The model under review builds one solid part; all positions refer to its coordinate system, in mm. A direction names the side the tool comes from. Coordinates: 2 decimals unless noted, no trailing zeros. Order: outer loops, then holes, each group sorted by start corner. A loop starts at its lowest first (then second) coordinate and runs counter-clockwise, first axis right, second up. Notation, with made-up numbers: (-0.75, 50) -> (16.25, 50) arc R28 ccw to (16.25, 74) -> close; hole circle Ø7 at (47, -18). An arc over 180 degrees is marked (long way). Use one line per item in the form item = value. Start each with the question number.
(1) Take a section at D-D (y = 3.75). State the section outline as (x, z) points.
(2) For faces 5 (the flat face through (0, 4.75, -19)), 6 (the flat face through (2.715, 9.521, -15.653)), 7 (the cylindrical face through (16.39, 10.1, -17.49)), list the 3-axis set-ups (+Z, -Z, +X, -X, +Y, -Y) from which the entire face can be reached by the end or side of a thin tool; tool diameter is ignored.
(3) Take a section at B-B (z = -27.25). State the section outline as (x, y) points.
(4) Insertion check: pin 1 Ø3.5 at (x, z) = (0, -17.25) entering from -Y; pin 2 Ø4 at (x, z) = (0, -17.25) entering from -Y; pin 3 Ø3.5 at (x, y) = (-10, -3.75) entering from +Z. Each pin has a flat end and moves straight along its axis. Give the tip position at first contact, or say it passes through.
(5) Wall thickness on line 1 along Y through (x, z) = (4, -18.5); line 2 along Y through (x, z) = (-2, -27.25); line 3 along Y through (x, z) = (-14.5, -22): over which ranges is each line inside the solid? List them lowest first.
(6) Mouldability with a two-part tool opening along Y and no side actions: class faces 1 (the cylindrical face through (0.241, 3.632, -30.248)), 2 (the flat face through (0, 0, -34.5)), 3 (the flat face through (2, 8, -17)), 4 (the cylindrical face through (-16.35, -10.14, -17.49)) as +Y half, -Y half, draft (parallel to the pull), parting line (faces both ways), or undercut.
(7) Take a section at A-A (x = -10). State the section outline as (y, z) points, then the cut area to 3 significant figures.
(8) Take a section at C-C (x = 0). State how many separate pieces and enclosed holes the cut face has, then the cut area to 3 significant figures.
```python
from build123d import *

# Parameters (mm, degrees)
SKETCH1_W           = 34.5
SKETCH1_H           = 22
BOSS_EXTRUDE1_DEPTH = 34.5
SKETCH2_R           = 3
CUT_EXTRUDE1_DEPTH  = 51.014997751
SKETCH3_R           = 1.5
CUT_EXTRUDE2_DEPTH  = 3
SKETCH3_3_R         = 1.5
CUT_EXTRUDE3_DEPTH  = 45.405095428
CHAMFER1_SIZE       = 2
FILLET1_R           = 3


with BuildPart() as part:
    # Sketch1 → Boss-Extrude1 (new body)
    with BuildSketch(Plane.XY):
        Rectangle(SKETCH1_W, SKETCH1_H)
        with BuildLine():
            ThreePointArc((-7.171572875, -4.75), (-13, -3.75), (-7.171572875, -2.75))
            Line((-7.171572875, -2.75), (7.171572875, -2.75))
            ThreePointArc((7.171572875, -2.75), (10.507305936, -0.793204321), (13, -3.75))
            ThreePointArc((13, -3.75), (10.507305936, -6.706795679), (7.171572875, -4.75))
            Line((7.171572875, -4.75), (-7.171572875, -4.75))
        make_face(mode=Mode.SUBTRACT)
    extrude(amount=-BOSS_EXTRUDE1_DEPTH)

    # Sketch2 → Cut-Extrude1 (cut, through all)
    with BuildSketch(Plane(origin=(17.25, 0, 0), x_dir=(0, 0, -1), z_dir=(1, 0, 0))):
        with Locations((7.25, 3.75)):
            Circle(SKETCH2_R)
        with BuildLine():
            Line((10.078427125, 2.75), (24.421572875, 2.75))
            ThreePointArc((24.421572875, 2.75), (24.25, 3.75), (24.421572875, 4.75))
            Line((24.421572875, 4.75), (10.078427125, 4.75))
            ThreePointArc((10.078427125, 4.75), (10.206795679, 4.257305936), (10.25, 3.75))
            ThreePointArc((10.25, 3.75), (10.206795679, 3.242694064), (10.078427125, 2.75))
        make_face()
        with Locations((27.25, 3.75)):
            Circle(SKETCH2_R)
    extrude(amount=-CUT_EXTRUDE1_DEPTH, mode=Mode.SUBTRACT)

    # Sketch3 → Cut-Extrude2 (cut)
    # profile 1 of 2: a face of its own
    with BuildSketch(Plane(origin=(0, 11, 0), x_dir=(1, 0, 0), z_dir=(0, 1, 0))):
        Polygon((3.637306696, 17.25), (1.818653348, 20.4), (-1.818653348, 20.4), (-3.637306696, 17.25), (-1.818653348, 14.1), (1.818653348, 14.1), align=None)
        with Locations((0, 17.25)):
            Circle(SKETCH3_R, mode=Mode.SUBTRACT)
    # profile 2 of 2: a face of its own
    with BuildSketch(Plane(origin=(0, 11, 0), x_dir=(1, 0, 0), z_dir=(0, 1, 0))):
        with Locations((0, 17.25)):
            Circle(SKETCH3_R)
    extrude(amount=-CUT_EXTRUDE2_DEPTH, mode=Mode.SUBTRACT)

    # Sketch3_3 → Cut-Extrude3 (cut, through all)
    with BuildSketch(Plane(origin=(0, 11, 0), x_dir=(1, 0, 0), z_dir=(0, 1, 0))):
        with Locations(Location((0, 17.25, 0), (0, 0, 270))):
            Circle(SKETCH3_3_R)
    extrude(amount=-CUT_EXTRUDE3_DEPTH, mode=Mode.SUBTRACT)

    # Chamfer1
    chamfer1_edges = [part.edges().sort_by_distance(p)[0] for p in [
        (0, -11, -18.75),
    ]]
    chamfer(chamfer1_edges, length=CHAMFER1_SIZE)

    # Fillet1
    fillet1_edges = [part.edges().sort_by_distance(p)[0] for p in [
        (17.25, -11, -17.25),
        (-17.25, -11, -17.25),
        (-17.25, 11, -17.25),
        (17.25, 11, -17.25),
    ]]
    fillet(fillet1_edges, radius=FILLET1_R)


solid = part.part
```
Findings:
q1.outline = (-17.25, -34.5) -> (17.25, -34.5) -> (17.25, -30.25) -> (-17.25, -30.25) -> close; (-17.25, -4.25) -> (17.25, -4.25) -> (17.25, 0) -> (-17.25, 0) -> close
q2.face_5 = +X, -X
q2.face_6 = +Y
q2.face_7 = +Z, -Z, +X, +Y
q3.outline = (-17.25, -8) arc R3 ccw to (-14.25, -11) -> (14.25, -11) arc R3 ccw to (17.25, -8) -> (17.25, 0.75) -> (-17.25, 0.75) -> close; (-17.25, 6.75) -> (17.25, 6.75) -> (17.25, 8) arc R3 ccw to (14.25, 11) -> (-14.25, 11) arc R3 ccw to (-17.25, 8) -> close; hole (-7.17, -4.75) -> (7.17, -4.75) arc R3 ccw (long way) to (7.17, -2.75) -> (-7.17, -2.75) arc R3 ccw (long way) to start
q4.pin_1 = -9.25
q4.pin_2 = -9.5
q4.pin_3 = through
q5.line_1 = -11 to -4.75, -2.75 to 2.75, 4.75 to 11
q5.line_2 = -11 to -4.75, -2.75 to 0.75, 6.75 to 11
q5.line_3 = -10.99 to 2.75, 4.75 to 10.99
q6.face_1 = undercut
q6.face_2 = draft
q6.face_3 = +Y half
q6.face_4 = -Y half
q7.outline = (-11, -34.5) -> (-6.75, -34.5) -> (-6.75, 0) -> (-11, 0) -> close; (-0.75, -34.5) -> (11, -34.5) -> (11, 0) -> (-0.75, 0) -> close; hole (2.75, -24.42) arc R3 ccw (long way) to (4.75, -24.42) -> (4.75, -10.08) arc R3 ccw (long way) to (2.75, -10.08) -> close
q7.area = 467 mm²
q8.separate_pieces = 4
q8.enclosed_holes = 0
q8.area = 537 mm²
